Check sheet for the modelled part. Datum: model origin and axes. Units: mm. Round coordinates to 2 decimals unless told otherwise and drop trailing zeros. Write each loop counter-clockwise with the first axis right and the second up, starting at its lowest first coordinate (ties: lowest second). Pieces come first, ordered by that corner, then holes. Notation, with made-up numbers: (67, 34.25) -> (102, 34.25) arc R32 ccw to (102, 66.25) -> close; hole circle Ø10 at (37, -36). An arc over 180 degrees is marked (long way). Write item = value, one per line.
Autodesk Inventor part; units mm, degrees
ref_plane "YZ Plane" through (0, 0, 0) normal (1, 0, 0) x (0, 1, 0)
ref_plane "XZ Plane" through (0, 0, 0) normal (0, 1, 0) x (-1, 0, 0)
ref_plane "XY Plane" through (0, 0, 0) normal (0, 0, 1) x (1, 0, 0)
sketch "Náčrt1" plane through (0, 0, 0) normal (1, 0, 0) x (0, 1, 0)
  line L0 (1.5, 0) -> (21.5, 0)
  line L1 (23, -1.5) -> (23, -21.5)
  line L2 (21.5, -23) -> (1.5, -23)
  line L3 (0, -21.5) -> (0, -1.5)
  arc A0 (23, -1.5) -> (21.5, 0) centre (21.5, -1.5) ccw
  arc A1 (21.5, -23) -> (23, -21.5) centre (21.5, -21.5) ccw
  arc A2 (0, -21.5) -> (1.5, -23) centre (1.5, -21.5) ccw
  arc A3 (1.5, 0) -> (0, -1.5) centre (1.5, -1.5) ccw
  circle A4 centre (21.5, -1.5) radius 1
  circle A5 centre (1.5, -21.5) radius 1
  circle A6 centre (1.5, -1.5) radius 1
  circle A7 centre (21.5, -21.5) radius 1
  point P0 (0, 0)
  point P1 (23, 0)
  point P2 (0, -23)
  dimension "d0" = 23
  dimension "d1" = 23
  dimension "d2" = 1.5
  dimension "d3" = 1.5
  dimension "d4" = 2
  dimension "d5" = 2
  dimension "d6" = 2
  dimension "d7" = 2
extrude "Vysunutí1" add sketch "Náčrt1" along normal blind 3
properties part number "HGLRC Micro 13A 4in1 BLHeli_S"
(1) Sectioned sample at A-A on x = 2.7. Enter the section's corners in (y, z), then the cut area to 3 significant figures.
Worked answers:
outline = (0, -21.5) arc R1.5 ccw to (1.5, -23) -> (21.5, -23) arc R1.5 ccw to (23, -21.5) -> (23, -1.5) arc R1.5 ccw to (21.5, 0) -> (1.5, 0) arc R1.5 ccw to (0, -1.5) -> close; hole circle Ø2 at (1.5, -21.5); hole circle Ø2 at (1.5, -1.5); hole circle Ø2 at (21.5, -21.5); hole circle Ø2 at (21.5, -1.5)
area = 515 mm²
(2) Material ranges on L1, parallel to Z at x = 1.2, y = 21.5; L2, parallel to Y at x = 2.85, z = -2.25; L3, parallel to Z at x = 2.65, y = 1, recorded low to high. Write a range as [from, to].
Worked answers:
L1 = [-23, -22.5], [-20.5, -2.5], [-0.5, 0]
L2 = [0, 0.84], [2.16, 20.84], [22.16, 23]
L3 = [-22.91, -22.37], [-20.63, -2.37], [-0.63, -0.09]
(3) Release check for a two-part mould opening along Y. For faces 1 (the flat face through (1, 12, -23)), 2 (the cylindrical face through (1.479, 1.283, -20.524)), 3 (the flat face through (1, 23, -11)) record: pulls with the +Y half, pulls with the -Y half, needs draft (parallel to the pull), parting line crosses it, or undercut.
Worked answers:
face_1 = needs draft
face_2 = undercut
face_3 = pulls with the +Y half
